The listing builds one solid part. Answer for the finished solid, in the listing's coordinates (mm). Face numbers are marked on the shaded views. A direction names the side the tool comes from. Give positions to 0.01 mm unless a question says otherwise; leave off trailing zeros. Write each loop counter-clockwise with the first axis right and the second up, starting at its lowest first coordinate (ties: lowest second). Pieces come first, ordered by that corner, then holes. Notation, with made-up numbers: (-9, -27.5) - (31, -27.5) arc R20 ccw to (31, -20.5) - close; hole circle Ø5 at (-8.5, 82). An arc over 180 degrees is marked (long way). Return JSON: item names as keys, results as strings.
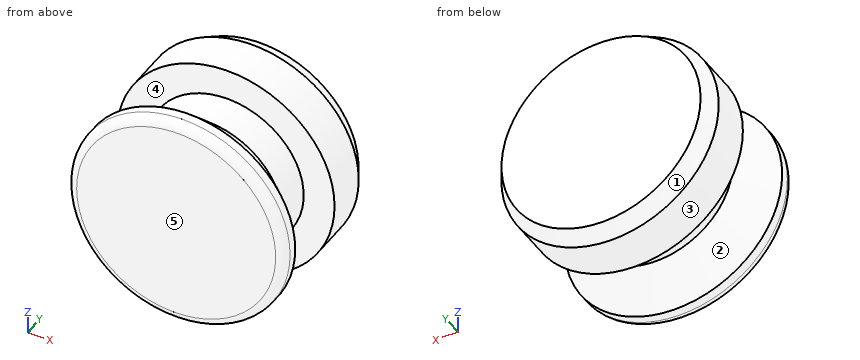
from build123d import *

# Parameters (mm, degrees)
FILLET1_R      = 0.79375
CHAMFER1_SIZE  = 0.79375
CHAMFER1_SIZE2 = 1.374815329


with BuildPart() as part:
    # Sketch1 → Revolve1 (revolve)
    with BuildSketch(Plane.XY):
        Polygon((0, 0), (-9.398, 0), (-9.398, 1.5875), (-6.731, 4.445), (-6.731, 7.62), (-9.398, 7.62), (-9.398, 12.7), (0, 12.7), align=None)
    revolve(axis=Axis((0, 0, 0), (0, 1, 0)))

    # Fillet1
    fillet1_edges = [part.edges().sort_by_distance(p)[0] for p in [
        (9.398, 0, 0),
    ]]
    fillet(fillet1_edges, radius=FILLET1_R)

    # Chamfer1
    chamfer1_edges = [part.edges().sort_by_distance(p)[0] for p in [
        (9.398, 12.7, 0),
    ]]
    chamfer1_side = [part.faces().sort_by_distance(p)[0] for p in [
        (0, 12.7, 0),
    ]]
    chamfer(chamfer1_edges, length=CHAMFER1_SIZE, length2=CHAMFER1_SIZE2, reference=chamfer1_side[0])


solid = part.part
Item 1: For the marked faces 1 and 2, determine the directions among +Z, -Z, +X, -X, +Y, -Y from which every point of the face is accessible in a straight line to the end or side of a thin tool.
Answer below:
{"face 1": "+Y", "face 2": "none"}
Item 2: Consider L1, parallel to Y at x = -6.75, z = 1.5; L2, parallel to Y at x = -5.75, z = 5.5; L3, parallel to Z at x = -1.5, y = 6.75. Determine where each line is inside the solid, lowest interval first.
Answer below:
{"L1": "y = 0 to 4.25, 7.62 to 12.7", "L2": "y = 0 to 3.13, 7.62 to 12.7", "L3": "z = -6.56 to 6.56"}
Item 3: A cutting plane is placed at A-A on x = 0. Determine the outline of the cut face in (y, z) (1 decimal).
Answer below:
{"outline": "(0, -8.6) arc R0.8 ccw to (0.8, -9.4) - (1.6, -9.4) - (4.4, -6.7) - (7.6, -6.7) - (7.6, -9.4) - (11.3, -9.4) - (12.7, -8.6) - (12.7, 8.6) - (11.3, 9.4) - (7.6, 9.4) - (7.6, 6.7) - (4.4, 6.7) - (1.6, 9.4) - (0.8, 9.4) arc R0.8 ccw to (0, 8.6) - close"}
Item 4: A cutting plane is placed at C-C on y = 9. Determine the outline of the cut face in (x, z), then the cut area to 3 significant figures.
Answer below:
{"outline": "circle Ø18.8 at (0, 0)", "area": "277 mm²"}
Item 5: The mould has two halves that part along Y. Classify the marked faces 3, 4 and 5: +Y half, -Y half, draft (parallel to the pull), parting line (faces both ways), or undercut.
Answer below:
{"face 3": "draft", "face 4": "undercut", "face 5": "-Y half"}
Item 6: A cutting plane is placed at B-B on z = 0. Determine the outline of the cut face in (x, y) (1 decimal).
Answer below:
{"outline": "(-9.4, 0.8) arc R0.8 ccw to (-8.6, 0) - (8.6, 0) arc R0.8 ccw to (9.4, 0.8) - (9.4, 1.6) - (6.7, 4.4) - (6.7, 7.6) - (9.4, 7.6) - (9.4, 11.3) - (8.6, 12.7) - (-8.6, 12.7) - (-9.4, 11.3) - (-9.4, 7.6) - (-6.7, 7.6) - (-6.7, 4.4) - (-9.4, 1.6) - close"}
Item 7: Flat-ended cylindrical pins translate along their axes: P1, Ø1.5, axis at x = -5.5, y = 1.5, coming from the +Z side; P2, Ø3, axis at x = 6, y = 8.5, coming from the -Z side; P3, Ø1, axis at y = 8.5, z = 5, coming from the -X side; P4, Ø4, axis at x = 0, z = 5, coming from the -Y side. Find the tip coordinate at first contact, or state that the pin passes through.
Answer below:
{"P1": "stops at z = 8.11", "P2": "stops at z = -8.25", "P3": "stops at x = -8.25", "P4": "stops at y = 0"}
